Input: dimensioned drawing with shaded views. Units: mm. Origin: part minimum x, y, z. A direction names the side the tool comes from. Round coordinates to 2 decimals unless told otherwise and drop trailing zeros. Write each loop counter-clockwise with the first axis right and the second up, starting at its lowest first coordinate (ties: lowest second). Pieces come first, ordered by that corner, then holes. Notation, with made-up numbers: M -35,7 L 18,7 A14 cw 18,15 Z; hole C 61,66 d1. An arc over 180 degrees is marked long. Use one line per item in the form item = value. Start each with the question number.
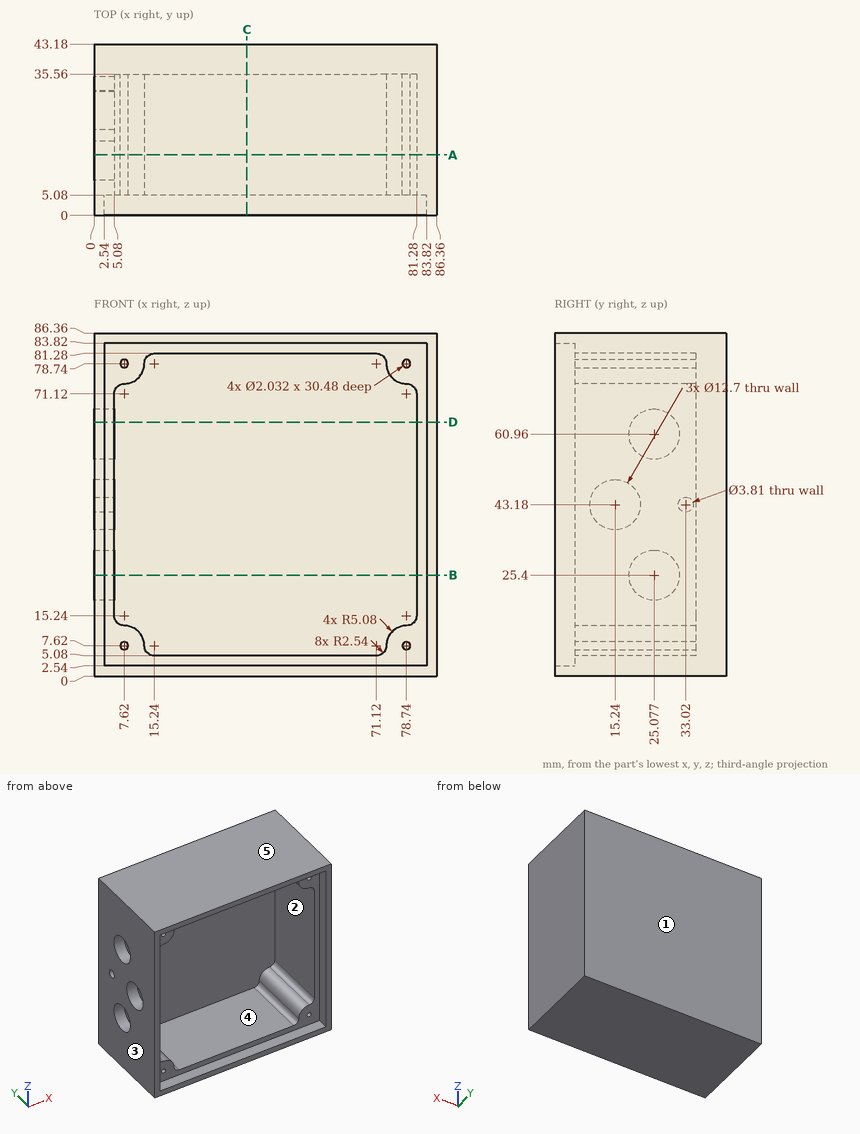
1. Pull-direction query (X, two-part tool) for the marked faces 3, 4 and 5; classes: released by +X, released by -X, zero draft, split by the parting line, or undercut.
2. Section query C-C (x = 38.5). Return loops of the section in (y, z).
3. Ray query, probe 1 along X at (y, z) = (14.5, 7.62); probe 2 along Z at (x, y) = (15, 2); probe 3 along Z at (x, y) = (44.5, 7). Return the intervals inside material, ascending.
4. Section query B-B (z = 25.4). Return loops of the section in (x, y).
5. Section query D-D (z = 64). Return loops of the section in (x, y).
6. Section query A-A (y = 15.24). Return loops of the section in (x, z).
7. Contact query for flat-ended pins moving along their axis: pin 1 (6 mm diameter, centred on x = 57, y = 38.5, fed in from -Z); pin 2 (1 mm diameter, centred on x = 7.5, z = 78.5, fed in from -Y); pin 3 (1.6 mm diameter, centred on x = 78.5, z = 79, fed in from -Y). Output: stop coordinate, or through.
8. Set-up query: the marked faces 1 and 2. Return all of +Z, -Z, +X, -X, +Y, -Y with unobstructed straight access to the full face (end or side cutting, diameter ignored); none if empty.
Checks:
q1.face_3 = released by -X
q1.face_4 = undercut
q1.face_5 = zero draft
q2.outline = M 0,0 L 43.18,0 L 43.18,86.36 L 0,86.36 L 0,83.82 L 5.08,83.82 L 5.08,81.28 L 35.56,81.28 L 35.56,5.08 L 5.08,5.08 L 5.08,2.54 L 0,2.54 Z
q3.probe_1 = 0 to 6.6, 8.64 to 12.7, 73.66 to 77.72, 79.76 to 86.36
q3.probe_2 = 0 to 2.54, 83.82 to 86.36
q3.probe_3 = 0 to 5.08, 81.28 to 86.36
q4.outline = M 0,0 L 2.54,0 L 2.54,5.08 L 5.08,5.08 L 5.08,18.73 L 0,18.73 Z; M 0,31.43 L 5.08,31.43 L 5.08,35.56 L 81.28,35.56 L 81.28,5.08 L 83.82,5.08 L 83.82,0 L 86.36,0 L 86.36,43.18 L 0,43.18 Z
q5.outline = M 0,0 L 2.54,0 L 2.54,5.08 L 5.08,5.08 L 5.08,19.5 L 0,19.5 Z; M 0,30.65 L 5.08,30.65 L 5.08,35.56 L 81.28,35.56 L 81.28,5.08 L 83.82,5.08 L 83.82,0 L 86.36,0 L 86.36,43.18 L 0,43.18 Z
q6.outline = M 0,0 L 86.36,0 L 86.36,86.36 L 0,86.36 L 0,49.53 L 5.08,49.53 L 5.08,71.12 A2.54 cw 7.62,73.66 A5.08 ccw 12.7,78.74 A2.54 cw 15.24,81.28 L 71.12,81.28 A2.54 cw 73.66,78.74 A5.08 ccw 78.74,73.66 A2.54 cw 81.28,71.12 L 81.28,15.24 A2.54 cw 78.74,12.7 A5.08 ccw 73.66,7.62 A2.54 cw 71.12,5.08 L 15.24,5.08 A2.54 cw 12.7,7.62 A5.08 ccw 7.62,12.7 A2.54 cw 5.08,15.24 L 5.08,36.83 L 0,36.83 Z; hole C 7.62,7.62 d2.03; hole C 7.62,78.74 d2.03; hole C 78.74,7.62 d2.03; hole C 78.74,78.74 d2.03
q7.pin_1 = 0
q7.pin_2 = 35.56
q7.pin_3 = 5.08
q8.face_1 = +Z, -Z, +X, -X, +Y
q8.face_2 = -Y
